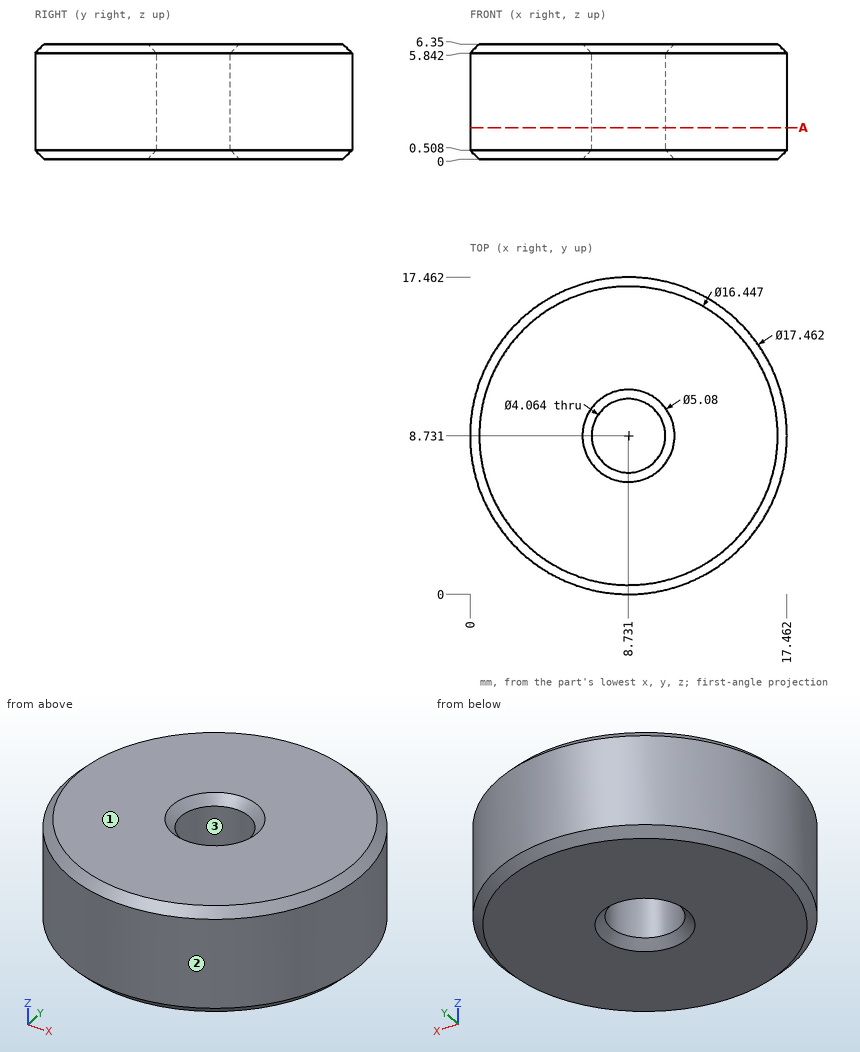
Print and shaded views of the part. All mm, measured from the part's lowest x, y and z. Coordinates: 2 decimals unless noted, no trailing zeros. Order: outer loops, then holes, each group sorted by start corner. A loop starts at its lowest first (then second) coordinate and runs counter-clockwise, first axis right, second up. Notation, with made-up numbers: (7, -40) - (47, -40) arc R15 cw to (47, -26) - close; hole circle Ø4 at (13.5, 67.25). An arc over 180 degrees is marked (long way). Put each result on its own line as item: value.
1. Saw through at A-A (z = 1.75). Write the cut outline in (x, y) (1 decimal).
Answer sheet:
outline: circle Ø17.5 at (8.7, 8.7); hole circle Ø4.1 at (8.7, 8.7)
2. Drop flat-ended pins along their axis: P1, Ø4.5, axis at x = 8.73, y = 8.73, coming from the +Z side; P2, Ø6, axis at x = 12.5, y = 2.5, coming from the -Z side; P3, Ø2, axis at x = 14, z = 2, coming from the +Y side; P4, Ø2, axis at x = 7, z = 1.5, coming from the -Y side. Give the stop position or say it passes through.
Answer sheet:
P1: stops at z = 6.06
P2: stops at z = 0
P3: stops at y = 16.35
P4: stops at y = 0.03
3. Pull direction X, two halves, no side cores. Call the marked faces 1, 2 and 3: pulls with the +X half, pulls with the -X half, needs draft (parallel to the pull), parting line crosses it, or undercut.
Answer sheet:
face 1: needs draft
face 2: parting line crosses it
face 3: undercut
4. Probe line 1 along X through (y, z) = (8, 5.5) (1 decimal); line 2 along Y through (x, z) = (10.5, 4) (1 decimal); line 3 along Y through (x, z) = (10.25, 1.5) (1 decimal). List the from-to ranges inside material, lowest first. Write a range as [from, to].
Answer sheet:
line 1: x = [0, 6.8], [10.6, 17.4]
line 2: y = [0.2, 7.7], [9.7, 17.3]
line 3: y = [0.1, 7.4], [10.1, 17.3]
